from build123d import *

# Parameters (mm, degrees)
CYLINDER264_R     = 2
CYLINDER264_DEPTH = 12
CYLINDER265_R     = 2
CYLINDER265_DEPTH = 12
BOX423_W          = 25
BOX423_H          = 10
BOX423_DEPTH      = 12
BOX424_W          = 25
BOX424_H          = 10
BOX424_DEPTH      = 12
BOX425_W          = 10
BOX425_H          = 20.4
BOX425_DEPTH      = 12
BOX426_W          = 10
BOX426_H          = 20.4
BOX426_DEPTH      = 12
BOX422_W          = 81.6
BOX422_H          = 10
BOX422_DEPTH      = 4
FILLET010_R       = 4.99
FILLET011_R       = 4.99
FILLET012_R       = 3
FILLET013_R       = 2


with BuildPart() as cylinder264:
    # Cylinder264 → Cylinder264 (new body)
    with BuildSketch(Plane(origin=(1.4, 70, 0), x_dir=(1, 0, 0), z_dir=(0, 0, 1))):
        Circle(CYLINDER264_R)
    extrude(amount=CYLINDER264_DEPTH)


with BuildPart() as fusion270:
    # Cylinder265 → Cylinder265 (new body)
    with BuildSketch(Plane(origin=(-70.2, 70, 0), x_dir=(1, 0, 0), z_dir=(0, 0, 1))):
        Circle(CYLINDER265_R)
    extrude(amount=CYLINDER265_DEPTH)

    # Fusion270: union Cylinder264
    add(cylinder264.part)


with BuildPart() as box423:
    # Box423 → Box423 (new body)
    with BuildSketch(Plane(origin=(-75.2, 65, 0), x_dir=(1, 0, 0), z_dir=(0, 0, 1))):
        with Locations((12.5, 5)):
            Rectangle(BOX423_W, BOX423_H)
    extrude(amount=BOX423_DEPTH)


with BuildPart() as box424:
    # Box424 → Box424 (new body)
    with BuildSketch(Plane(origin=(-18.6, 65, 0), x_dir=(1, 0, 0), z_dir=(0, 0, 1))):
        with Locations((12.5, 5)):
            Rectangle(BOX424_W, BOX424_H)
    extrude(amount=BOX424_DEPTH)


with BuildPart() as box425:
    # Box425 → Box425 (new body)
    with BuildSketch(Plane(origin=(-60.2, 54.6, 0), x_dir=(1, 0, 0), z_dir=(0, 0, 1))):
        with Locations((5, 10.2)):
            Rectangle(BOX425_W, BOX425_H)
    extrude(amount=BOX425_DEPTH)


with BuildPart() as box426:
    # Box426 → Box426 (new body)
    with BuildSketch(Plane(origin=(-18.6, 54.6, 0), x_dir=(1, 0, 0), z_dir=(0, 0, 1))):
        with Locations((5, 10.2)):
            Rectangle(BOX426_W, BOX426_H)
    extrude(amount=BOX426_DEPTH)


with BuildPart() as cut414:
    # Box422 → Box422 (new body)
    with BuildSketch(Plane(origin=(-75.2, 65, 0), x_dir=(1, 0, 0), z_dir=(0, 0, 1))):
        with Locations((40.8, 5)):
            Rectangle(BOX422_W, BOX422_H)
    extrude(amount=BOX422_DEPTH)

    # Fusion269: union Box423, Box424, Box425, Box426
    add(box423.part)
    add(box424.part)
    add(box425.part)
    add(box426.part)

    # Fillet010
    fillet010_edges = [cut414.edges().sort_by_distance(p)[0] for p in [
        (-75.2, 65, 8),
        (-75.2, 75, 8),
    ]]
    fillet(fillet010_edges, radius=FILLET010_R)

    # Fillet011
    fillet011_edges = [cut414.edges().sort_by_distance(p)[0] for p in [
        (6.4, 75, 8),
        (6.4, 65, 8),
    ]]
    fillet(fillet011_edges, radius=FILLET011_R)

    # Fillet012
    fillet012_edges = [cut414.edges().sort_by_distance(p)[0] for p in [
        (-8.6, 54.6, 6),
        (-18.6, 54.6, 6),
        (-50.2, 54.6, 6),
        (-60.2, 54.6, 6),
    ]]
    fillet(fillet012_edges, radius=FILLET012_R)

    # Fillet013
    fillet013_edges = [cut414.edges().sort_by_distance(p)[0] for p in [
        (-34.4, 65, 4),
        (-34.4, 75, 4),
    ]]
    fillet(fillet013_edges, radius=FILLET013_R)

    # Cut414: cut Fusion270
    add(fusion270.part, mode=Mode.SUBTRACT)


solid = cut414.part
Design review of the part built by this model. Coordinates are the model's own, in mm. A direction names the side the tool comes from. Round coordinates to 2 decimals unless told otherwise and drop trailing zeros. Write each loop counter-clockwise with the first axis right and the second up, starting at its lowest first coordinate (ties: lowest second). Pieces come first, ordered by that corner, then holes. Notation, with made-up numbers: (10, 52.25) -> (22, 52.25) arc R28 ccw to (22, 83.25) -> close; hole circle Ø11 at (3.25, 52.5). An arc over 180 degrees is marked (long way). One line per item, written item: value. Start each with the question number.
Q1. The part is to be moulded in two halves that separate along Y. For faces 1 (the face through (4.899, 73.577, 6.084)), 2 (the face through (-9.46, 55.5, 6.08)), 3 (the face through (1.14, 71.983, 5.916)), say which applies: pulls with the +Y half, pulls with the -Y half, needs draft (parallel to the pull), parting line crosses it, or undercut.
Q2. Add section B-B (y = 59.25). Give the boundary of the cut face in (x, z), then the cut area to 3 significant figures.
Q3. Add section A-A (z = 5.5). State how many separate pieces and enclosed holes the cut face has, then the cut area to 3 significant figures.
Q4. Insertion check: P1, Ø5, axis at x = -31, y = 67, coming from the +Z side; P2, Ø3.5, axis at y = 62.5, z = 7.5, coming from the +X side; P3, Ø3, axis at x = -70.2, y = 70, coming from the +Z side; P4, Ø5, axis at y = 65.5, z = 6.5, coming from the -X side. Each pin has a flat end and moves straight along its axis. Give the tip position at first contact, or say it passes through.
Q5. Tool access review of faces 4 (the face through (-34.18, 74.43, 3.4)), 5 (the face through (-65, 65, 6)), 6 (the face through (-35, 65, 1)): name each direction out of +Z, -Z, +X, -X, +Y, -Y from which nothing blocks a thin tool from reaching the whole face with its end or side.
Q6. To check wall thickness, follow probe 1 along X at (y, z) = (64, 10.75); probe 2 along Y at (x, z) = (1.4, 4); probe 3 along Z at (x, y) = (-28.5, 69.5). State the ranges of each line that lie inside material, in increasing order.
Q7. Add section C-C (x = -32). Give the boundary of the cut face in (y, z).
Q8. Add section D-D (x = -61). Give the boundary of the cut face in (y, z).
Response:
1. face 1: pulls with the +Y half
1. face 2: pulls with the -Y half
1. face 3: undercut
2. outline: (-60.2, 0) -> (-50.2, 0) -> (-50.2, 12) -> (-60.2, 12) -> close; (-18.6, 0) -> (-8.6, 0) -> (-8.6, 12) -> (-18.6, 12) -> close
2. area: 240 mm^2
3. separate pieces: 2
3. enclosed holes: 2
3. area: 654 mm^2
4. P1: stops at z = 4
4. P2: stops at x = -8.6
4. P3: passes through
4. P4: stops at x = -74.79
5. face 4: +Z, +Y
5. face 5: +Z, -Z, -X, -Y
5. face 6: +Z, -Z, -Y
6. probe 1: x = -60.2 to -50.2, -18.6 to -8.6
6. probe 2: y = 65 to 68, 72 to 75
6. probe 3: z = 0 to 4
7. outline: (65, 0) -> (75, 0) -> (75, 2) arc R2 ccw to (73, 4) -> (67, 4) arc R2 ccw to (65, 2) -> close
8. outline: (65, 0) -> (75, 0) -> (75, 12) -> (65, 12) -> close
